The listing builds one solid part. Answer for the finished solid, in the listing's coordinates (mm). Face numbers are marked on the shaded views. A direction names the side the tool comes from. Coordinates: 2 decimals unless noted, no trailing zeros. Write each loop counter-clockwise with the first axis right and the second up, starting at its lowest first coordinate (ties: lowest second). Pieces come first, ordered by that corner, then holes.
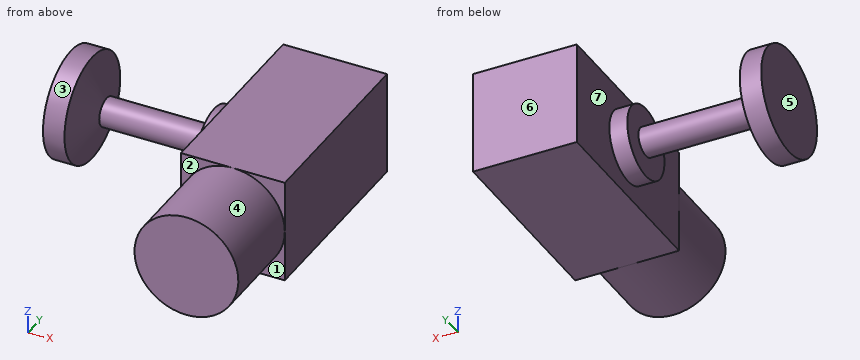
from build123d import *

# Parameters (mm, degrees)
SKETCH_2_W      = 29
SKETCH_2_H      = 55
EXTRUDE_1_DEPTH = 29
SKETCH_3_R      = 14.5
EXTRUDE_2_DEPTH = 25


with BuildPart() as part:
    # 草图1 → 旋转3 (revolve)
    with BuildSketch(Plane.XY, mode=Mode.PRIVATE) as revolve_3_sk:
        Polygon((-10, 15), (-10, 0), (35, 0), (35, 10), (30, 10), (30, 4), (0, 4), (-4, 15), align=None)
    revolve(revolve_3_sk.sketch.rotate(Axis((-10, 0, 0), (1, 0, 0)), 90), axis=Axis((-10, 0, 0), (1, 0, 0)))

    # 草图2 → 凸台-拉伸1 (add)
    with BuildSketch(Plane(origin=(35, 0, 0), x_dir=(0, 0, -1), z_dir=(1, 0, 0))):
        Rectangle(SKETCH_2_W, SKETCH_2_H)
    extrude(amount=EXTRUDE_1_DEPTH)

    # 草图3 → 凸台-拉伸2 (add)
    with BuildSketch(Plane.XZ.offset(27.5)):
        with Locations(Location((49.5, 0, 0), (0, 0, 270))):
            Circle(SKETCH_3_R)
    extrude(amount=EXTRUDE_2_DEPTH)


solid = part.part
Q1. The part is cut by section B-B, the plane x = 44.5. Write down the section's boundary in (y, z), then the cut area to 3 significant figures.
Answers below:
outline: (-52.5, -13.61) - (-27.5, -13.61) - (-27.5, -14.5) - (27.5, -14.5) - (27.5, 14.5) - (-27.5, 14.5) - (-27.5, 13.61) - (-52.5, 13.61) - close
area: 2,280 mm2
Q2. Determine the mould class of the marked faces 4, 5, 6 and 7 for opening direction X: released by +X, released by -X, zero draft, split by the parting line, or undercut.
Answers below:
face 4: split by the parting line
face 5: released by -X
face 6: zero draft
face 7: undercut
Q3. Which of the six approach directions +Z, -Z, +X, -X, +Y, -Y give full straight-line access (tool end or side, diameter ignored) to the marked faces 1, 2 and 3?
Answers below:
face 1: -Z, +X, -Y
face 2: +Z, -X, -Y
face 3: -X
Q4. The part is cut by section C-C, the plane y = -46.5. Write down the section's boundary in (x, z).
Answers below:
outline: circle Ø29 at (49.5, 0)
Q5. The part is cut by section A-A, the plane y = 0. Write down the section's boundary in (x, z), then the cut area to 3 significant figures.
Answers below:
outline: (-10, -15) - (-4, -15) - (0, -4) - (30, -4) - (30, -10) - (35, -10) - (35, -14.5) - (64, -14.5) - (64, 14.5) - (35, 14.5) - (35, 10) - (30, 10) - (30, 4) - (0, 4) - (-4, 15) - (-10, 15) - close
area: 1,440 mm2
Q6. The part is cut by section D-D, the plane x = 3. Write down the section's boundary in (y, z).
Answers below:
outline: circle Ø8 at (0, 0)
Q7. Find the intervals of material crossed by probe 1 along X at (y, z) = (19, 2.75); probe 2 along Y at (x, z) = (41, -13.5); probe 3 along X at (y, z) = (-8, -8.5), in increasing order.
Answers below:
probe 1: x = 35 to 64
probe 2: y = -27.5 to 27.5
probe 3: x = -10 to -2.79, 35 to 64
Q8. Given pin 1 (10 mm diameter, centred on x = 31.5, y = -36.5, fed in from -Z); pin 2 (4 mm diameter, centred on x = 42, y = -4.5, fed in from -Z), each flat-ended and moving along its own axis, determine where each tip first touches the part or whether it passes through.
Answers below:
pin 1: stops at z = -6.42
pin 2: stops at z = -14.5
